from build123d import *

# Parameters (mm, degrees)
F1_DEPTH = 350
F2_SIZE  = 3
F4_D     = 19
F6_D     = 3.3
F6_DEPTH = 14.1
F6_TIP   = 0.9914200214
F8_D     = 3.3
F8_DEPTH = 14.1
F8_TIP   = 0.9914200214


with BuildPart() as f1:
    # F0 (on Front) → F1 (new body)
    with BuildSketch(Plane.XZ):
        Polygon((2, 17.25), (-3, 17.25), (-3, -17.25), (2, -17.25), (2, -20.25), (-3, -20.25), (-3, -21.6), (5, -21.6), (5, 21.6), (-3, 21.6), (-3, 20.25), (2, 20.25), align=None)
    extrude(amount=F1_DEPTH)

    # F2
    f2_edges = [f1.edges().sort_by_distance(p)[0] for p in [
        (5, -175, -21.6),
        (5, -175, 21.6),
    ]]
    chamfer(f2_edges, length=F2_SIZE)

    # F4 (through all)
    with Locations(Plane.YZ.offset(5)):
        with Locations((-25, 0)):
            Hole(F4_D / 2)

    # F6
    with Locations(Plane(origin=(0, 0, 0), x_dir=(1, 0, 0), z_dir=(0, 1, 0))):
        with Locations((1, -11.28), (1, 11.28)):
            Hole(F6_D / 2, depth=F6_DEPTH)
            with Locations((0, 0, -(F6_DEPTH + F6_TIP / 2))):  # 118° drill point
                Cone(0, F6_D / 2, F6_TIP, mode=Mode.SUBTRACT)

    # F8
    with Locations(Plane.XZ.offset(350)):
        with Locations((1, 14.1), (1, -14.1)):
            Hole(F8_D / 2, depth=F8_DEPTH)
            with Locations((0, 0, -(F8_DEPTH + F8_TIP / 2))):  # 118° drill point
                Cone(0, F8_D / 2, F8_TIP, mode=Mode.SUBTRACT)


solid = f1.part
Work out the finished part from the listing and answer in its coordinate system (mm). Give positions to 0.01 mm unless a question says otherwise; leave off trailing zeros. Loops run counter-clockwise (first coordinate to the right, second up) from the corner with the lowest first, then second, coordinate; pieces in that order, holes last. Notation, with made-up numbers: (5.25, 5) - (28.25, 5) arc R20 ccw to (28.25, 16) - close; hole circle Ø7 at (-21, -32). An arc over 180 degrees is marked (long way). Answer in a Markdown table with one row per item.
(1) Section B-B (y = -65.5) is taken. Give the vertices of the cut face in (x, z), and give its area (3 significant figures).
Results list:
| item | result |
|---|---|
| outline | (-3, -21.6) - (2, -21.6) - (5, -18.6) - (5, 18.6) - (2, 21.6) - (-3, 21.6) - (-3, 20.25) - (2, 20.25) - (2, 17.25) - (-3, 17.25) - (-3, -17.25) - (2, -17.25) - (2, -20.25) - (-3, -20.25) - close |
| area | 307 mm² |
(2) For a pull along Y with two mould halves and no side action, classify faces 1 (the face through (1, 0, 0)), 2 (the face through (0.94, -15.51, 0.42)), 3 (the face through (5, -173, 0)) as pulls with the +Y half, pulls with the -Y half, needs draft (parallel to the pull), parting line crosses it, or undercut.
Results list:
| item | result |
|---|---|
| face 1 | pulls with the +Y half |
| face 2 | undercut |
| face 3 | needs draft |
(3) Section A-A (z = 0) is taken. Give the vertices of the cut face in (x, y).
Results list:
| item | result |
|---|---|
| outline | (-3, -350) - (5, -350) - (5, -34.5) - (-3, -34.5) - close; (-3, -15.5) - (5, -15.5) - (5, 0) - (-3, 0) - close |
(4) Section C-C (y = -30.5) is taken. Give the vertices of the cut face in (x, z).
Results list:
| item | result |
|---|---|
| outline | (-3, -21.6) - (2, -21.6) - (5, -18.6) - (5, -7.75) - (-3, -7.75) - (-3, -17.25) - (2, -17.25) - (2, -20.25) - (-3, -20.25) - close; (-3, 7.75) - (5, 7.75) - (5, 18.6) - (2, 21.6) - (-3, 21.6) - (-3, 20.25) - (2, 20.25) - (2, 17.25) - (-3, 17.25) - close |
(5) Consider L1, parallel to Z at x = -1, y = -292.5; L2, parallel to Z at x = 1, y = -340; L3, parallel to Z at x = 1, y = -3. Determine where each line is inside the solid, lowest interval first. Write a range as [from, to].
Results list:
| item | result |
|---|---|
| L1 | z = [-21.6, -20.25], [-17.25, 17.25], [20.25, 21.6] |
| L2 | z = [-21.6, -20.25], [-17.25, -15.75], [-12.45, 12.45], [15.75, 17.25], [20.25, 21.6] |
| L3 | z = [-21.6, -20.25], [-17.25, -12.93], [-9.63, 9.63], [12.93, 17.25], [20.25, 21.6] |
(6) Flat-ended cylindrical pins translate along their axes: pin 1 Ø0.9 at (y, z) = (-255.5, 19.5) entering from -X; pin 2 Ø3 at (x, z) = (1, -11.28) entering from +Y. Find the tip coordinate at first contact, or state that the pin passes through.
Results list:
| item | result |
|---|---|
| pin 1 | stops at x = 2 |
| pin 2 | stops at y = -14.19 |
